The listing builds one solid part. Answer for the finished solid, in the listing's coordinates (mm). A direction names the side the tool comes from. Round coordinates to 2 decimals unless told otherwise and drop trailing zeros. Write each loop counter-clockwise with the first axis right and the second up, starting at its lowest first coordinate (ties: lowest second). Pieces come first, ordered by that corner, then holes. Notation, with made-up numbers: (52, 33.5) - (108, 33.5) arc R10 cw to (108, 51.5) - close; hole circle Ø4 at (41.25, 23). An arc over 180 degrees is marked (long way). Use a Markdown table: item, result. Add a question column.
1) A cutting plane is placed at C-C (z = 14.5). Give the vertices of the cut face in (x, y).
2) A tool of negligible diameter and unlimited length cuts with its end or side. For faces 1 (the cylindrical face through (-14.4, -4.4, -64.1)), 2 (the cylindrical face through (-8.324, -7.638, 71.334)), from which of +Z, -Z, +X, -X, +Y, -Y can it reach the whole face along a straight path? Write none if from no direction.
3) A cutting plane is placed at D-D (y = -2.75). Give the vertices of the cut face in (x, z) (3 decimals).
4) A cutting plane is placed at A-A (x = 12.7). Give the vertices of the cut face in (y, z), then the cut area to 3 significant figures.
5) Find the intervals of material crossed by probe 1 along Z at (x, y) = (0, -7.9); probe 2 along Z at (x, y) = (-17.5, -7.25); probe 3 along Y at (x, z) = (-45, 10.5), in increasing order. Write a range as from..to.
6) Determine the mould class of faces 3 (the cylindrical face through (-60.47, -4.383, -46.367)), 4 (the flat face through (-1, -6.35, 9)), 5 (the flat face through (-6, -8.89, -56)) for opening direction X: +X half, -X half, draft (parallel to the pull), parting line (faces both ways), or undercut.
7) A cutting plane is placed at B-B (x = 28). Give the vertices of the cut face in (y, z), then the cut area to 3 significant figures.
8) Each of these flat-tipped pins is pushed along its axis until it touches: P1, Ø1.5, axis at x = 42.5, y = -2, coming from the +Z side; P2, Ø5, axis at x = -28.5, y = -1, coming from the -Z side; P3, Ø10, axis at x = 12.7, z = -66.57, coming from the -Y side; P4, Ø5, axis at x = 24.5, z = -32.5, coming from the -Y side. Where does it stop, or does it pass through?
```python
from build123d import *

# Parameters (mm, degrees)
F0_R     = 76.2
F1_DEPTH = 8.89
F2_R     = 63.9445
F3_DEPTH = 2.54
F5_D     = 6.35


with BuildPart() as f1:
    # F0 (on Front) → F1 (new body)
    with BuildSketch(Plane.XZ):
        Circle(F0_R)
    extrude(amount=F1_DEPTH)

    # F2 (on face) → F3 (cut)
    with BuildSketch(Plane.XZ.offset(8.89)):
        with Locations((0, 7.933864)):
            Circle(F2_R)
    extrude(amount=-F3_DEPTH, mode=Mode.SUBTRACT)

    # F5 (through all)
    with Locations(Plane.XZ.offset(8.89)):
        with Locations((-12.699133, -66.782228), (12.7, -66.572319)):
            Hole(F5_D / 2)


solid = f1.part
```
Entries:
| question | item | result |
|---|---|---|
| 1 | outline | (-74.81, -8.89) - (-63.61, -8.89) - (-63.61, -6.35) - (63.61, -6.35) - (63.61, -8.89) - (74.81, -8.89) - (74.81, 0) - (-74.81, 0) - close |
| 2 | face 1 | +Y, -Y |
| 2 | face 2 | -Y |
| 3 | outline | circle Ø152.4 at (0, 0); hole circle Ø6.35 at (-12.699, -66.782); hole circle Ø6.35 at (12.7, -66.572) |
| 4 | outline | (-8.89, -75.13) - (0, -75.13) - (0, -69.75) - (-8.89, -69.75) - close; (-8.89, -63.4) - (0, -63.4) - (0, 75.13) - (-8.89, 75.13) - (-8.89, 70.6) - (-6.35, 70.6) - (-6.35, -54.74) - (-8.89, -54.74) - close |
| 4 | area | 961 mm² |
| 5 | probe 1 | z = -76.2..-56.01, 71.88..76.2 |
| 5 | probe 2 | z = -74.16..-53.57, 69.44..74.16 |
| 5 | probe 3 | y = -6.35..0 |
| 6 | face 3 | parting line |
| 6 | face 4 | undercut |
| 6 | face 5 | draft |
| 7 | outline | (-8.89, -70.87) - (0, -70.87) - (0, 70.87) - (-8.89, 70.87) - (-8.89, 65.42) - (-6.35, 65.42) - (-6.35, -49.55) - (-8.89, -49.55) - close |
| 7 | area | 968 mm² |
| 8 | P1 | stops at z = 63.74 |
| 8 | P2 | stops at z = -71.63 |
| 8 | P3 | stops at y = -8.89 |
| 8 | P4 | stops at y = -6.35 |
